Autodesk Inventor part; units mm, degrees
ref_plane "YZ Plane" through (0, 0, 0) normal (1, 0, 0) x (0, 1, 0)
ref_plane "XZ Plane" through (0, 0, 0) normal (0, 1, 0) x (-1, 0, 0)
ref_plane "XY Plane" through (0, 0, 0) normal (0, 0, 1) x (1, 0, 0)
sketch "Sketch1" plane through (0, 0, 0) normal (0, 0, 1) x (1, 0, 0)
  line L0 (-70, -7.5) -> (70, -7.5)
  line L1 (70, -7.5) -> (70, 7.5)
  line L2 (70, 7.5) -> (-70, 7.5)
  line L3 (-70, 7.5) -> (-70, -7.5)
  line L4 (-70, -7.5) -> (70, 7.5) construction
  line L5 (70, -7.5) -> (-70, 7.5) construction
  circle A0 centre (0, 0) radius 15
  line L6 (-73.4722, 0) -> (96.5278, 0) construction
  circle A1 centre (-60, 0) radius 2.75
  line L7 (0, 0) -> (0, 31) construction
  circle A2 centre (60, 0) radius 2.75
  circle A3 centre (0, 0) radius 1.5
  circle A4 centre (-6.9148, 6.9148) radius 1.7526
  line L8 (0, 0) -> (-14.5685, 14.5685) construction
  circle A5 centre (-6.9148, -6.9148) radius 1.7526
  circle A6 centre (6.9148, -6.9148) radius 1.7526
  circle A7 centre (6.9148, 6.9148) radius 1.7526
  point P0 (0, 0)
  dimension "d0" = 140
  dimension "d1" = 15
  dimension "d4" = 30
  dimension "d5" = 5.5
  dimension "d6" = 10
  dimension "d10" = 3
  dimension "d11" = 3.5052
  dimension "d12" = 45
  dimension "d13" = 6.9148
  dimension "d16" = 360
extrude "Extrusion1" add sketch "Sketch1" along normal blind 4 contours L3 L2 A0 L0 | A0 L2 A4 A7 L0 A6 A5 | L0 A5 A6 A0 | A5 L0 | L0 A5 | A0 L2 A7 A4 | A0 L2 L1 L0 | A4 L2 | L2 A4 | A6 L0 | L0 A6 | A7 L2 | L2 A7 | A1 | A2 | A3
extrude "Extrusion2" cut sketch "Sketch1" along normal through all contours A5 L0 | L0 A5 | A4 L2 | L2 A4 | A6 L0 | L0 A6 | A7 L2 | L2 A7 | A1 | A2 | A3
fillet "Fillet1" radius 5 4 edges at (70, -7.5, 2) (70, 7.5, 2) (-70, -7.5, 2) (-70, 7.5, 2)
equation "\"BendRadius\" = Thickness"
equation "\"BendReliefWidth\" = Thickness"
equation "\"BendReliefDepth\" = 0.5 * Thickness"
equation "\"CornerReliefSize\" = 4 * Thickness"
equation "\"MinimumRemnant\" = 2 * Thickness"
equation "\"TransitionRadius\" = BendRadius"
equation "\"JacobiRadiusSize\" = Thickness"
equation "\"GapSize\" = Thickness"
properties part number "rudder_horn"
Verification items for the finished model (mm, model axes). A direction names the side the tool comes from. Round coordinates to 2 decimals unless told otherwise and drop trailing zeros. Order: outer loops, then holes, each group sorted by start corner. A loop starts at its lowest first (then second) coordinate and runs counter-clockwise, first axis right, second up. Notation, with made-up numbers: (2, -15.5) -> (41, -15.5) arc R21 cw to (41, -3.5) -> close; hole circle Ø6 at (76.25, -24). An arc over 180 degrees is marked (long way). Put each result on its own line as item: value.
1) Section check C-C (z = 3.35). Record the cut outline in (x, y).
Final values:
outline: (-70, -2.5) arc R5 ccw to (-65, -7.5) -> (-12.99, -7.5) arc R15 ccw to (12.99, -7.5) -> (65, -7.5) arc R5 ccw to (70, -2.5) -> (70, 2.5) arc R5 ccw to (65, 7.5) -> (12.99, 7.5) arc R15 ccw to (-12.99, 7.5) -> (-65, 7.5) arc R5 ccw to (-70, 2.5) -> close; hole circle Ø5.5 at (-60, 0); hole circle Ø3.51 at (-6.91, -6.91); hole circle Ø3.51 at (-6.91, 6.91); hole circle Ø3 at (0, 0); hole circle Ø3.51 at (6.91, -6.91); hole circle Ø3.51 at (6.91, 6.91); hole circle Ø5.5 at (60, 0)
2) Mould release check, pull along Y, two halves, no side actions. Record for faces 1 (the flat face through (70, 0, 2)), 2 (the cylindrical face through (6.535, 8.626, 1.972)), 3 (the cylindrical face through (68.5, -6.07, 2.03)): +Y half, -Y half, draft (parallel to the pull), parting line (faces both ways), or undercut.
Final values:
face 1: draft
face 2: undercut
face 3: -Y half
3) Section check A-A (y = 0). Record the cut outline in (x, z).
Final values:
outline: (-70, 0) -> (-62.75, 0) -> (-62.75, 4) -> (-70, 4) -> close; (-57.25, 0) -> (-1.5, 0) -> (-1.5, 4) -> (-57.25, 4) -> close; (1.5, 0) -> (57.25, 0) -> (57.25, 4) -> (1.5, 4) -> close; (62.75, 0) -> (70, 0) -> (70, 4) -> (62.75, 4) -> close
4) Depth check by flat-ended pin: pin 1 (2 mm diameter, centred on x = 35, z = 2.5, fed in from -Y); pin 2 (2 mm diameter, centred on x = 49.5, z = 2.5, fed in from +Y). Enter the tip coordinate at first touch or a pass-through.
Final values:
pin 1: stops at y = -7.5
pin 2: stops at y = 7.5
5) Material ranges on line 1 (X direction, y = 0, z = 1.55); line 2 (Y direction, x = -60, z = 2.1); line 3 (X direction, y = -0.5, z = 0.9), recorded low to high.
Final values:
line 1: x = -70 to -62.75, -57.25 to -1.5, 1.5 to 57.25, 62.75 to 70
line 2: y = -7.5 to -2.75, 2.75 to 7.5
line 3: x = -70 to -62.7, -57.3 to -1.41, 1.41 to 57.3, 62.7 to 70
6) Section check B-B (x = -60). Record the cut outline in (y, z).
Final values:
outline: (-7.5, 0) -> (-2.75, 0) -> (-2.75, 4) -> (-7.5, 4) -> close; (2.75, 0) -> (7.5, 0) -> (7.5, 4) -> (2.75, 4) -> close
7) Section check D-D (x = -43.5). Record the cut outline in (y, z), then the cut area to 3 significant figures.
Final values:
outline: (-7.5, 0) -> (7.5, 0) -> (7.5, 4) -> (-7.5, 4) -> close
area: 60.0 mm^2
8) Set-up check for faces 4 (the flat face through (-39, 7.5, 2)), 5 (the flat face through (-39, -7.5, 2)), 6 (the flat face through (39, -7.5, 2)), 7 (the flat face through (39, 7.5, 2)): record each of +Z, -Z, +X, -X, +Y, -Y from which the full face is reachable in a straight line by a thin tool's end or side.
Final values:
face 4: +Z, -Z, -X, +Y
face 5: +Z, -Z, -X, -Y
face 6: +Z, -Z, +X, -Y
face 7: +Z, -Z, +X, +Y
